Here's how the part is built. I have some questions about the finished solid (model axes, mm). A direction names the side the tool comes from. Coordinates: 2 decimals unless noted, no trailing zeros. Write each loop counter-clockwise with the first axis right and the second up, starting at its lowest first coordinate (ties: lowest second). Pieces come first, ordered by that corner, then holes. Notation, with made-up numbers: (62, 27.5) -> (116, 27.5) arc R18 ccw to (116, 55.5) -> close; hole circle Ø10 at (85.5, 44.25). An arc over 180 degrees is marked (long way). Use a Markdown table: item, result. Add a question column.
Item 1: Imagine slicing it at C-C, the plane z = 2. Write out the boundary of the cut face in (x, y).
Item 2: If I drill on line 1 along Y through (x, z) = (0, 3.5); line 2 along X through (y, z) = (-15.75, 5.5); line 3 along X through (y, z) = (-8.5, 3.5), over which ranges is the centre line in solid material (lowest first)? Write a range as from..to.
Item 3: On a 3-axis mill with a long thin cutter (end or side, diameter ignored), from which of +Z, -Z, +X, -X, +Y, -Y can I reach the whole of each face in a straight line? I mean faces 1 (the flat face through (9, -12.7, 3)), 2 (the cylindrical face through (0, 0, 3)), 3 (the flat face through (-10, -12.7, 3)). Say none if no direction works.
Item 4: Will this pin go through, and if not, where does the flat tip stop? pin 1 Ø3.5 at (x, y) = (0, -7.94) entering from -Z.
Item 5: Imagine slicing it at B-B, the plane y = -8.75. Write out the boundary of the cut face in (x, z).
Item 6: Imagine slicing it at A-A, the plane x = 0. Write out the boundary of the cut face in (y, z).
Item 7: Imagine slicing it at D-D, the plane y = -13.5. Write out the boundary of the cut face in (x, z).
```python
from build123d import *

# Parameters (mm, degrees)
BASE_DEPTH          = 6.35
AXLE_HOLE_D         = 4.3053
SKETCH8_W           = 12.7
SKETCH8_H           = 6.35
BOSS_EXTRUDE2_DEPTH = 6.35


with BuildPart() as part:
    # Sketch1 → Base (new body)
    with BuildSketch(Plane.XY):
        with BuildLine():
            Line((-12.7, -12.7), (12.7, -12.7))
            ThreePointArc((12.7, -12.7), (0, 0), (-12.7, -12.7))
        make_face()
    extrude(amount=BASE_DEPTH)

    # Axle hole (through all)
    with Locations(Plane(origin=(0, 0, 0), x_dir=(-1, 0, 0), z_dir=(0, 0, -1))):
        with Locations((0, -7.9375)):
            Hole(AXLE_HOLE_D / 2)

    # Sketch8 → Boss-Extrude2 (add)
    with BuildSketch(Plane.XY.offset(6.35)):
        with Locations((0, -15.875)):
            Rectangle(SKETCH8_W, SKETCH8_H)
    extrude(amount=-BOSS_EXTRUDE2_DEPTH)


solid = part.part
```
Ans:
| question | item | result |
|---|---|---|
| 1 | outline | (-12.7, -12.7) -> (-6.35, -12.7) -> (-6.35, -19.05) -> (6.35, -19.05) -> (6.35, -12.7) -> (12.7, -12.7) arc R12.7 ccw to start; hole circle Ø4.31 at (0, -7.94) |
| 2 | line 1 | y = -19.05..-10.09, -5.78..0 |
| 2 | line 2 | x = -6.35..6.35 |
| 2 | line 3 | x = -11.99..-2.08, 2.08..11.99 |
| 3 | face 1 | +Z, -Z, +X, -Y |
| 3 | face 2 | +Z, -Z, +Y |
| 3 | face 3 | +Z, -Z, -X, -Y |
| 4 | pin 1 | passes through |
| 5 | outline | (-12.07, 0) -> (-1.99, 0) -> (-1.99, 6.35) -> (-12.07, 6.35) -> close; (1.99, 0) -> (12.07, 0) -> (12.07, 6.35) -> (1.99, 6.35) -> close |
| 6 | outline | (-19.05, 0) -> (-10.09, 0) -> (-10.09, 6.35) -> (-19.05, 6.35) -> close; (-5.78, 0) -> (0, 0) -> (0, 6.35) -> (-5.78, 6.35) -> close |
| 7 | outline | (-6.35, 0) -> (6.35, 0) -> (6.35, 6.35) -> (-6.35, 6.35) -> close |
